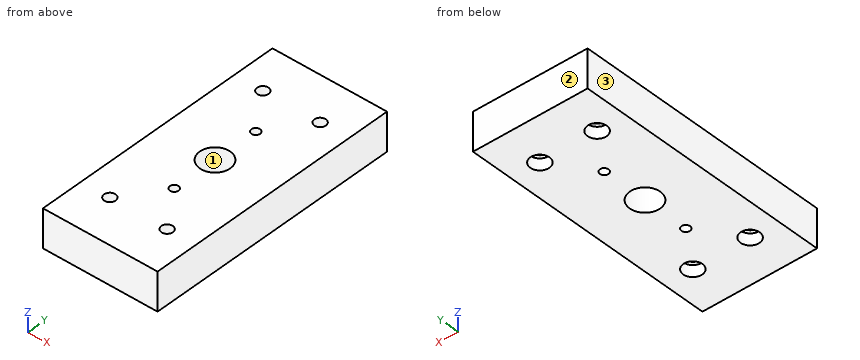
from build123d import *

# Parameters (mm, degrees)
SKETCH1_R          = 3
SKETCH1_R_2        = 2.25
EXTRUDE1_DEPTH     = 20
SKETCH2_R          = 5
CUT_EXTRUDE1_DEPTH = 6
SKETCH3_R          = 8
CUT_EXTRUDE2_DEPTH = 20
SKETCH4_W          = 10
SKETCH4_H          = 135
EXTRUDE2_DEPTH     = 20


with BuildPart() as part:
    # Sketch1 → Extrude1 (new body)
    with BuildSketch(Plane.XY):
        Polygon((5, 135), (0, 135), (-10, 135), (-10, 0), (0, 0), (40, 0), (50, 0), (50, 135), (40, 135), align=None)
        with Locations((5, 22.5)):
            Circle(SKETCH1_R, mode=Mode.SUBTRACT)
        with Locations((35, 22.5)):
            Circle(SKETCH1_R, mode=Mode.SUBTRACT)
        with Locations((20.000131027, 43.499934589)):
            Circle(SKETCH1_R_2, mode=Mode.SUBTRACT)
        with Locations((5, 112.5)):
            Circle(SKETCH1_R, mode=Mode.SUBTRACT)
        with Locations((20.000131027, 91.49994372)):
            Circle(SKETCH1_R_2, mode=Mode.SUBTRACT)
        with Locations((35, 112.5)):
            Circle(SKETCH1_R, mode=Mode.SUBTRACT)
    extrude(amount=EXTRUDE1_DEPTH)

    # Sketch2 → Cut-Extrude1 (cut)
    with BuildSketch(Plane(origin=(0, 0, 0), x_dir=(-1, 0, 0), z_dir=(0, 0, -1))):
        with Locations((-35, 112.5)):
            Circle(SKETCH2_R)
        with Locations((-5, 112.5)):
            Circle(SKETCH2_R)
        with Locations((-35, 22.5)):
            Circle(SKETCH2_R)
        with Locations((-5, 22.5)):
            Circle(SKETCH2_R)
    extrude(amount=-CUT_EXTRUDE1_DEPTH, mode=Mode.SUBTRACT)

    # Sketch3 → Cut-Extrude2 (cut)
    with BuildSketch(Plane(origin=(0, 0, 0), x_dir=(-1, 0, 0), z_dir=(0, 0, -1))):
        with Locations((-20, 67.5)):
            Circle(SKETCH3_R)
    extrude(amount=-CUT_EXTRUDE2_DEPTH, mode=Mode.SUBTRACT)

    # Sketch4 → Extrude2 (add)
    with BuildSketch(Plane(origin=(0, 0, 0), x_dir=(-1, 0, 0), z_dir=(0, 0, -1))):
        with Locations((-45, 67.5)):
            Rectangle(SKETCH4_W, SKETCH4_H)
        with Locations((5, 67.5)):
            Rectangle(SKETCH4_W, SKETCH4_H)
    extrude(amount=-EXTRUDE2_DEPTH)


solid = part.part
For this review, take the finished solid that the model builds, in its own axes (mm). Face numbers are marked on the shaded views. Round coordinates to 2 decimals unless told otherwise and drop trailing zeros. Order: outer loops, then holes, each group sorted by start corner. A loop starts at its lowest first (then second) coordinate and runs counter-clockwise, first axis right, second up. Notation, with made-up numbers: (-10.5, 16) -> (29.5, 16) arc R27 ccw to (29.5, 55) -> close; hole circle Ø8 at (-30, 1). An arc over 180 degrees is marked (long way). Write item = value, one per line. Start each with the question number.
1) The part is to be moulded in two halves that separate along Y. For the marked faces 1, 2 and 3, say which applies: +Y half, -Y half, draft (parallel to the pull), parting line (faces both ways), or undercut.
2) Take a section at A-A on y = 112.5. State the section outline as (x, z) points.
3) Take a section at D-D on x = 20. State the section outline as (y, z) points, plus the area to 3 significant figures.
4) To check wall thickness, follow line 1 (Y direction, x = 5, z = 4.25); line 2 (Y direction, x = 35, z = 17); line 3 (Y direction, x = 20.5, z = 15.5). State the ranges of each line that lie inside material, in increasing order. Write a range as from..to.
5) Take a section at B-B on y = 67.5. State the section outline as (x, z) points, plus the area to 3 significant figures.
6) Insertion check: pin 1 (11 mm diameter, centred on x = 34.5, y = 20, fed in from -Z); pin 2 (3.5 mm diameter, centred on x = 35, y = 22.5, fed in from -Z); pin 3 (5 mm diameter, centred on x = 34, y = 114.5, fed in from -Z). Each pin has a flat end and moves straight along its axis. Give the tip position at first contact, or say it passes through.
7) Take a section at C-C on x = 35. State the section outline as (y, z) points.
Verdict:
q1.face_1 = undercut
q1.face_2 = +Y half
q1.face_3 = draft
q2.outline = (-10, 0) -> (0, 0) -> (0, 6) -> (2, 6) -> (2, 20) -> (-10, 20) -> close; (8, 6) -> (10, 6) -> (10, 0) -> (30, 0) -> (30, 6) -> (32, 6) -> (32, 20) -> (8, 20) -> close; (38, 6) -> (40, 6) -> (40, 0) -> (50, 0) -> (50, 20) -> (38, 20) -> close
q3.outline = (0, 0) -> (41.25, 0) -> (41.25, 20) -> (0, 20) -> close; (45.75, 0) -> (59.5, 0) -> (59.5, 20) -> (45.75, 20) -> close; (75.5, 0) -> (89.25, 0) -> (89.25, 20) -> (75.5, 20) -> close; (93.75, 0) -> (135, 0) -> (135, 20) -> (93.75, 20) -> close
q3.area = 2,200 mm2
q4.line_1 = 0..17.5, 27.5..107.5, 117.5..135
q4.line_2 = 0..19.5, 25.5..109.5, 115.5..135
q4.line_3 = 0..41.31, 45.69..59.52, 75.48..89.31, 93.69..135
q5.outline = (-10, 0) -> (12, 0) -> (12, 20) -> (-10, 20) -> close; (28, 0) -> (50, 0) -> (50, 20) -> (28, 20) -> close
q5.area = 880 mm2
q6.pin_1 = 0
q6.pin_2 = through
q6.pin_3 = 6
q7.outline = (0, 0) -> (17.5, 0) -> (17.5, 6) -> (19.5, 6) -> (19.5, 20) -> (0, 20) -> close; (25.5, 6) -> (27.5, 6) -> (27.5, 0) -> (107.5, 0) -> (107.5, 6) -> (109.5, 6) -> (109.5, 20) -> (25.5, 20) -> close; (115.5, 6) -> (117.5, 6) -> (117.5, 0) -> (135, 0) -> (135, 20) -> (115.5, 20) -> close
